Input: part model. Units: mm. Frame: model coordinates. Give positions to 0.01 mm unless a question says otherwise; leave off trailing zeros. Order: outer loops, then holes, each group sorted by start corner. A loop starts at its lowest first (then second) coordinate and runs counter-clockwise, first axis right, second up. Notation, with made-up numbers: M 72,82.5 L 123,82.5 A27 cw 123,118.5 Z; hole C -15.5,29 d6. An arc over 180 degrees is marked long. Use a Markdown table: item, result.
from build123d import *

# Parameters (mm, degrees)
F0_W     = 37.681248
F0_H     = 36.994756
F1_DEPTH = 1.6
F2_R     = 1
F3_DEPTH = 25


with BuildPart() as f1:
    # F0 (on Top) → F1 (new body)
    with BuildSketch(Plane.XY):
        Rectangle(F0_W, F0_H)
    extrude(amount=F1_DEPTH)

    # F2 (on face) → F3 (cut)
    with BuildSketch(Plane.XY.offset(1.6)):
        Circle(F2_R)
        with Locations((0, 15.2)):
            Circle(F2_R)
        with Locations((15.2, 0)):
            Circle(F2_R)
        with Locations((15.2, 15.2)):
            Circle(F2_R)
    extrude(amount=-F3_DEPTH, mode=Mode.SUBTRACT)


solid = f1.part
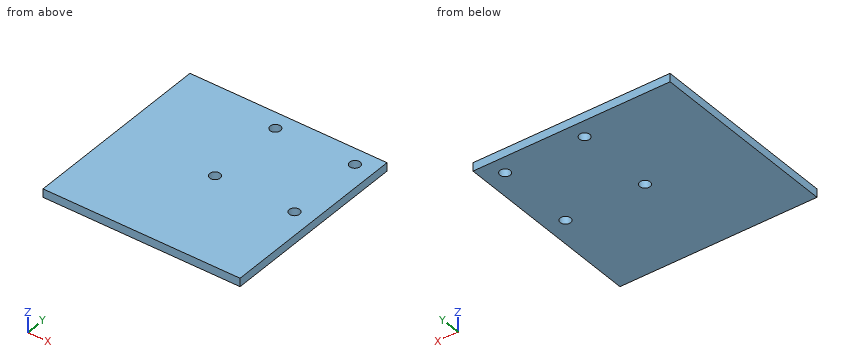
1) Material intervals for line 1 (Y direction, x = 15.2, z = 0.75), sorted ascending. Write a range as from..to.
Response values:
| item | result |
|---|---|
| line 1 | y = -18.5..-1, 1..14.2, 16.2..18.5 |
2) Cut plane B-B on x = 0. Return loops of the section in (y, z), and give its area (3 significant figures).
Response values:
| item | result |
|---|---|
| outline | M -18.5,0 L -1,0 L -1,1.6 L -18.5,1.6 Z; M 1,0 L 14.2,0 L 14.2,1.6 L 1,1.6 Z; M 16.2,0 L 18.5,0 L 18.5,1.6 L 16.2,1.6 Z |
| area | 52.8 mm² |
3) Cut plane A-A on y = 0. Return loops of the section in (x, z), and give its area (3 significant figures).
Response values:
| item | result |
|---|---|
| outline | M -18.84,0 L -1,0 L -1,1.6 L -18.84,1.6 Z; M 1,0 L 14.2,0 L 14.2,1.6 L 1,1.6 Z; M 16.2,0 L 18.84,0 L 18.84,1.6 L 16.2,1.6 Z |
| area | 53.9 mm² |
